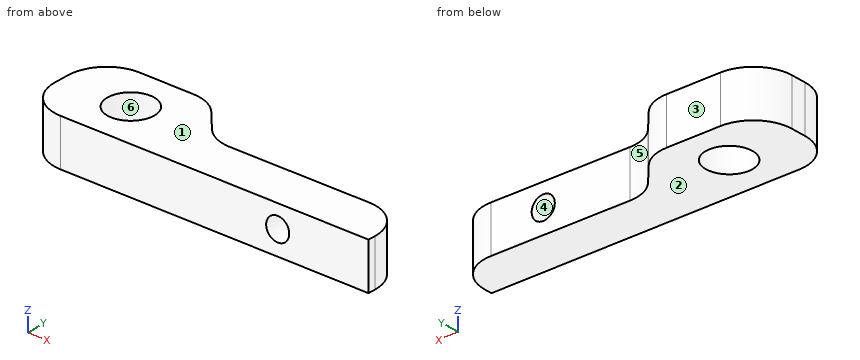
```python
from build123d import *

# Parameters (mm, degrees)
F0_R     = 3
F2_DEPTH = 6
F3_D     = 3
F4_R     = 5
F5_R     = 5
F6_R     = 5
F7_R     = 5


with BuildPart() as f2:
    # F0 (on Top) → F2 (new body)
    with BuildSketch(Plane.XY):
        Polygon((-19.694119, 12), (-19.694119, 0), (25.346741, 0), (25.346741, 6), (0, 5.890472), (-5.3996, 12), align=None)
        with Locations((-10.694119, 6)):
            Circle(F0_R, mode=Mode.SUBTRACT)
    extrude(amount=F2_DEPTH)

    # F3 (through all)
    with Locations(Plane.XZ):
        with Locations((13.534061, 3.085485)):
            Hole(F3_D / 2)

    # F4
    f4_edges = [f2.edges().sort_by_distance(p)[0] for p in [
        (-19.694119, 12, 3),
        (-19.694119, 0, 3),
    ]]
    fillet(f4_edges, radius=F4_R)

    # F5
    f5_edges = [f2.edges().sort_by_distance(p)[0] for p in [
        (-5.3996, 12, 3),
    ]]
    fillet(f5_edges, radius=F5_R)

    # F6
    f6_edges = [f2.edges().sort_by_distance(p)[0] for p in [
        (0, 5.890472, 3),
    ]]
    fillet(f6_edges, radius=F6_R)

    # F7
    f7_edges = [f2.edges().sort_by_distance(p)[0] for p in [
        (25.346741, 6, 3),
    ]]
    fillet(f7_edges, radius=F7_R)


solid = f2.part
```
Part model, mm, in its own coordinate system. Face numbers are marked on the shaded views. A direction names the side the tool comes from. Round coordinates to 2 decimals unless told otherwise and drop trailing zeros. Write each loop counter-clockwise with the first axis right and the second up, starting at its lowest first coordinate (ties: lowest second). Pieces come first, ordered by that corner, then holes. Notation, with made-up numbers: M -36.75,16.25 L 6.25,16.25 A24 ccw 6.25,26.25 Z; hole C 9.25,65 d3. An arc over 180 degrees is marked long. Answer as CSV lines item,"result". Start each with the question number.
1) Band-saw the part on A-A (z = 0.6). List the corners of the cut face in (x, y), then the cut area to 3 significant figures.
2) Which spindle directions (+Z, -Z, +X, -X, +Y, -Y) get a long thin tool onto all of the face, cutting with end or side? Do the marked faces 5 and 6. Say none if no direction does.
3) Mould opens along Z. For the marked faces 1, 2, 3 and 4 say: +Z half, -Z half, draft (parallel to the pull), parting line (faces both ways), or undercut.
4) Band-saw the part on C-C (x = 12.5). List the corners of the cut face in (y, z).
5) Drop flat-ended pins along their axis: pin 1 (3 mm diameter, centred on y = 3, z = 4, fed in from +X); pin 2 (3 mm diameter, centred on y = 7, z = 2.5, fed in from +X); pin 3 (1.5 mm diameter, centred on x = 14, y = 8.5, fed in from -Z); pin 4 (1 mm diameter, centred on y = 9.5, z = 3, fed in from +X). Give the stop position or say it passes through.
6) Drill centre lines: L1, parallel to Y at x = -15, z = 1.5; L2, parallel to Y at x = 19, z = 4.8; L3, parallel to X at y = 2.5, z = 2.45. Where is each one in solid material? Low to high.
7) Band-saw the part on B-B (y = 4). List the corners of the cut face in (x, z), then the cut area to 3 significant figures.
8) Band-saw the part on D-D (z = 3.6). List the corners of the cut face in (x, y).
Worked out:
1,outline,"M -19.69,5 A5 ccw -14.69,0 L 25.35,0 L 25.35,0.98 A5 ccw 20.33,5.98 L 2.27,5.9 A5 cw -1.5,7.59 L -3.91,10.31 A5 ccw -7.65,12 L -14.69,12 A5 ccw -19.69,7 Z; hole C -10.69,6 d6"
1,area,"326 mm²"
2,face 5,"+Z, -Z, +Y"
2,face 6,"+Z, -Z"
3,face 1,"+Z half"
3,face 2,"-Z half"
3,face 3,"draft"
3,face 4,"undercut"
4,outline,"M 0,0 L 5.94,0 L 5.94,2 L 0,2 Z; M 0,4.17 L 5.94,4.17 L 5.94,6 L 0,6 Z"
5,pin 1,"x = 25.32"
5,pin 2,"x = 22.48"
5,pin 3,"through"
5,pin 4,"x = -2.75"
6,L1,"0.01 to 11.99"
6,L2,"0 to 5.97"
6,L3,"-19.02 to 12.18, 14.89 to 25.11"
7,outline,"M -19.59,0 L -12.93,0 L -12.93,6 L -19.59,6 Z; M -8.46,0 L 24.33,0 L 24.33,6 L -8.46,6 Z; hole C 13.53,3.09 d3"
7,area,"230 mm²"
8,outline,"M -19.69,5 A5 ccw -14.69,0 L 12.13,0 L 12.13,5.94 L 2.27,5.9 A5 cw -1.5,7.59 L -3.91,10.31 A5 ccw -7.65,12 L -14.69,12 A5 ccw -19.69,7 Z; M 14.94,0 L 25.35,0 L 25.35,0.98 A5 ccw 20.33,5.98 L 14.94,5.96 Z; hole C -10.69,6 d6"
